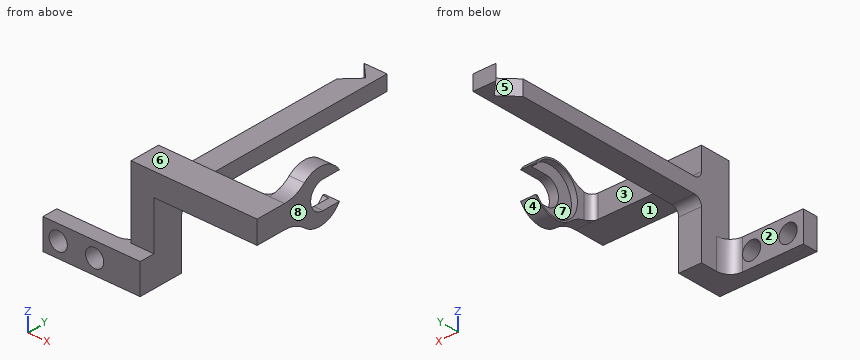
from build123d import *

# Parameters (mm, degrees)
SKETCH2_W                            = 22
SKETCH2_H                            = 10
SKETCH2_R                            = 3
BOSS_EXTRUDE1_DEPTH                  = 5
SKETCH3_W                            = 10
SKETCH3_H                            = 5
BOSS_EXTRUDE2_DEPTH                  = 10
BOSS_EXTRUDE3_DEPTH                  = 10
SKETCH5_W                            = 7.5
SKETCH5_H                            = 5
BOSS_EXTRUDE4_DEPTH                  = 75
CUT_EXTRUDE1_REACH                   = 98.857
BOSS_EXTRUDE5_DEPTH                  = 10
SKETCH13_W                           = 5
SKETCH13_H                           = 10
BOSS_EXTRUDE6_DEPTH                  = 7.5
BOSS_EXTRUDE7_DEPTH                  = 5
CUT_EXTRUDE5_REACH                   = 118.454
SKETCH16_R                           = 8
CUT_EXTRUDE6_DEPTH                   = 2
BOSS_EXTRUDE8_REACH                  = 104.314
BOSS_EXTRUDE8_END_RADIUS             = 11.091410312
BOSS_EXTRUDE8_DIRECTION_2_REACH      = 104.314
BOSS_EXTRUDE8_DIRECTION_2_END_RADIUS = 11.091410312
BOSS_EXTRUDE9_DEPTH                  = 7.5
BOSS_EXTRUDE10_START                 = -10
BOSS_EXTRUDE10_DEPTH                 = 10


with BuildPart() as part:
    # Sketch2 → Boss-Extrude1 (new body)
    with BuildSketch(Plane(origin=(0, 0, 0), x_dir=(1, 0, 0), z_dir=(0, 1, 0))):
        with Locations((6, 0)):
            Rectangle(SKETCH2_W, SKETCH2_H)
        with Locations(Location((0, 0, 0), (0, 0, 270))):
            Circle(SKETCH2_R, mode=Mode.SUBTRACT)
        with Locations(Location((12, 0, 0), (0, 0, 270))):
            Circle(SKETCH2_R, mode=Mode.SUBTRACT)
    extrude(amount=BOSS_EXTRUDE1_DEPTH)

    # Sketch3 → Boss-Extrude2 (add)
    with BuildSketch(Plane.XY.offset(5)):
        with Locations((22, 2.5)):
            Rectangle(SKETCH3_W, SKETCH3_H)
    extrude(amount=-BOSS_EXTRUDE2_DEPTH)

    # Sketch4 → Boss-Extrude3 (add)
    with BuildSketch(Plane(origin=(0, 5, 0), x_dir=(1, 0, 0), z_dir=(0, 1, 0))):
        Polygon((27, 5), (27, -5), (27, -7.5), (27, -18.5), (19.5, -18.5), (19.5, -7.5), (19.5, 5), align=None)
    extrude(amount=BOSS_EXTRUDE3_DEPTH)

    # Sketch5 → Boss-Extrude4 (add)
    with BuildSketch(Plane(origin=(0, 15, 0), x_dir=(1, 0, 0), z_dir=(0, 1, 0))):
        with Locations((23.25, -16)):
            Rectangle(SKETCH5_W, SKETCH5_H)
    extrude(amount=BOSS_EXTRUDE4_DEPTH)

    # Sketch6 → Cut-Extrude1 (cut, up to next)
    with BuildSketch(Plane.XY.offset(18.5), mode=Mode.PRIVATE) as cut_extrude1_sk1:
        Polygon((19.5, 90), (24.5, 85), (19.5, 80), align=None)
    cut_extrude1_tool1 = extrude(cut_extrude1_sk1.sketch, amount=-CUT_EXTRUDE1_REACH, mode=Mode.PRIVATE) & part.part
    add(cut_extrude1_tool1.solids().sort_by_distance((21.166667, 85, 18.5))[0], mode=Mode.SUBTRACT)

    # Sketch7 → Boss-Extrude5 (add)
    with BuildSketch(Plane(origin=(0, 15, 0), x_dir=(1, 0, 0), z_dir=(0, 1, 0))):
        Polygon((19.5, 5), (19.5, -28.5), (56, -28.5), (56, -21), (27, -21), (27, 5), align=None)
    extrude(amount=-BOSS_EXTRUDE5_DEPTH)

    # Sketch13 → Boss-Extrude6 (add)
    with BuildSketch(Plane(origin=(0, 0, 21), x_dir=(-1, 0, 0), z_dir=(0, 0, -1))):
        with Locations((-58.5, 10)):
            Rectangle(SKETCH13_W, SKETCH13_H)
    extrude(amount=-BOSS_EXTRUDE6_DEPTH)

    # Sketch14 → Boss-Extrude7 (add)
    with BuildSketch(Plane(origin=(61, 0, 0), x_dir=(0, 0, -1), z_dir=(1, 0, 0))):
        with BuildLine():
            Line((-29.25, 35), (-20.25, 35))
            ThreePointArc((-20.25, 35), (-16.346490099, 29.066011911), (-18.310852147, 22.240260236))
            ThreePointArc((-18.310852147, 22.240260236), (-20.306000981, 18.86176399), (-21, 15))
            Line((-21, 15), (-28.5, 15))
            ThreePointArc((-28.5, 15), (-29.193999019, 18.86176399), (-31.189147853, 22.240260236))
            ThreePointArc((-31.189147853, 22.240260236), (-33.153509901, 29.066011911), (-29.25, 35))
        make_face()
    extrude(amount=-BOSS_EXTRUDE7_DEPTH)

    # Sketch15 → Cut-Extrude5 (cut, up to next)
    with BuildSketch(Plane(origin=(61, 0, 0), x_dir=(0, 0, -1), z_dir=(1, 0, 0)), mode=Mode.PRIVATE) as cut_extrude5_sk1:
        with BuildLine():
            Line((-29.25, 35), (-29.25, 29))
            ThreePointArc((-29.25, 29), (-24.75, 24.5), (-20.25, 29))
            Line((-20.25, 29), (-20.25, 35))
            Line((-20.25, 35), (-29.25, 35))
        make_face()
    cut_extrude5_tool1 = extrude(cut_extrude5_sk1.sketch, amount=-CUT_EXTRUDE5_REACH, mode=Mode.PRIVATE) & part.part
    add(cut_extrude5_tool1.solids().sort_by_distance((61, 30.179951, 24.75))[0], mode=Mode.SUBTRACT)

    # Sketch16 → Cut-Extrude6 (cut)
    with BuildSketch(Plane(origin=(56, 0, 0), x_dir=(0, 0, -1), z_dir=(1, 0, 0))):
        with Locations((-24.75, 27.788897449)):
            Circle(SKETCH16_R)
    extrude(amount=CUT_EXTRUDE6_DEPTH, mode=Mode.SUBTRACT)

    # Boss-Extrude8: up to this cylinder (the profile starts outside it)
    boss_extrude8_end = Plane(origin=(55.44158, 15, 9.908589688), z_dir=(1, 0, 0)) * Cylinder(BOSS_EXTRUDE8_END_RADIUS, 231.810820624, mode=Mode.PRIVATE)
    # Sketch17 → Boss-Extrude8 (add, up to the surface)
    with BuildSketch(Plane(origin=(56, 15, 28.5), x_dir=(-1, 0, 0), z_dir=(0, 0, -1)), mode=Mode.PRIVATE) as boss_extrude8_sk1:
        with BuildLine():
            Line((0, 0), (0, 2.5))
            ThreePointArc((0, 2.5), (0.732233047, 0.732233047), (2.5, 0))
            Line((2.5, 0), (0, 0))
        make_face()
    boss_extrude8_tool1 = extrude(boss_extrude8_sk1.sketch, amount=BOSS_EXTRUDE8_REACH, mode=Mode.PRIVATE) - boss_extrude8_end
    add(boss_extrude8_tool1.solids().sort_by_distance((55.44158, 15.55842, 28.5))[0])

    # Boss-Extrude8 direction 2: up to this cylinder (the profile starts outside it)
    boss_extrude8_direction_2_end = Plane(origin=(55.44158, 15, 39.591410312), z_dir=(1, 0, 0)) * Cylinder(BOSS_EXTRUDE8_DIRECTION_2_END_RADIUS, 231.810820624, mode=Mode.PRIVATE)
    # Sketch17 → Boss-Extrude8 direction 2 (add, up to the surface)
    with BuildSketch(Plane(origin=(56, 15, 28.5), x_dir=(-1, 0, 0), z_dir=(0, 0, -1)), mode=Mode.PRIVATE) as boss_extrude8_direction_2_sk1:
        with BuildLine():
            Line((0, 0), (0, 2.5))
            ThreePointArc((0, 2.5), (0.732233047, 0.732233047), (2.5, 0))
            Line((2.5, 0), (0, 0))
        make_face()
    boss_extrude8_direction_2_tool1 = extrude(boss_extrude8_direction_2_sk1.sketch, amount=-BOSS_EXTRUDE8_DIRECTION_2_REACH, mode=Mode.PRIVATE) - boss_extrude8_direction_2_end
    add(boss_extrude8_direction_2_tool1.solids().sort_by_distance((55.44158, 15.55842, 28.5))[0])

    # Sketch18 → Boss-Extrude9 (add)
    with BuildSketch(Plane(origin=(27, 0, 0), x_dir=(0, 0, -1), z_dir=(1, 0, 0))):
        with BuildLine():
            Line((-13.5, 15), (-13.5, 17.5))
            ThreePointArc((-13.5, 17.5), (-12.767766953, 15.732233047), (-11, 15))
            Line((-11, 15), (-13.5, 15))
        make_face()
        with BuildLine():
            Line((-18.5, 15), (-18.5, 17.5))
            ThreePointArc((-18.5, 17.5), (-19.232233047, 15.732233047), (-21, 15))
            Line((-21, 15), (-18.5, 15))
        make_face()
    extrude(amount=-BOSS_EXTRUDE9_DEPTH)

    # Sketch19 → Boss-Extrude10 (add)
    with BuildSketch(Plane(origin=(0, 0, -5), x_dir=(-1, 0, 0), z_dir=(0, 0, -1)).offset(BOSS_EXTRUDE10_START)):
        with BuildLine():
            Line((-19.5, 5), (-19.5, 9.5))
            ThreePointArc((-19.5, 9.5), (-18.181980515, 6.318019485), (-15, 5))
            Line((-15, 5), (-19.5, 5))
        make_face()
    extrude(amount=BOSS_EXTRUDE10_DEPTH)


solid = part.part
Input: part model. Units: mm. Frame: model coordinates. Face numbers are marked on the shaded views. A direction names the side the tool comes from. Coordinates: 2 decimals unless noted, no trailing zeros. Loops run counter-clockwise (first coordinate to the right, second up) from the corner with the lowest first, then second, coordinate; pieces in that order, holes last.
(1) Section D-D on z = 24.75. Return the cut outline in (x, y), then the cut area to 3 significant figures.
(2) First-contact query: pin 1 Ø2.5 at (x, y) = (25, 52.5) entering from -Z; pin 2 Ø7.5 at (y, z) = (29.5, 28) entering from -X; pin 3 Ø6 at (x, z) = (24.5, 5) entering from +Y. Flat tips, straight axial feed; report the tip coordinate or a pass-through.
(3) Section C-C on x = 26. Return the cut outline in (y, z), then the cut area to 3 significant figures.
(4) Pull-direction query (X, two-part tool) for the marked faces 5, 6, 7 and 8; classes: released by +X, released by -X, zero draft, split by the parting line, or undercut.
(5) Set-up query: the marked faces 1, 2, 3 and 4. Return all of +Z, -Z, +X, -X, +Y, -Y with unobstructed straight access to the full face (end or side cutting, diameter ignored); none if empty.
(6) Section B-B on z = 1.5. Return the cut outline in (x, y), then the cut area to 3 significant figures.
(7) Section A-A on x = 12. Return the cut outline in (y, z), then the cut area to 3 significant figures.
(8) Material intervals for probe 1 along X at (y, z) = (2.45, 0); probe 2 along Z at (x, y) = (12, 2.1); probe 3 along Z at (x, y) = (40, 5.5), sorted ascending.
Data:
1. outline: (19.5, 5) - (61, 5) - (61, 24.5) - (58, 24.5) - (58, 19.79) - (56, 19.79) - (56, 17.5) arc R2.5 cw to (53.5, 15) - (19.5, 15) - close
1. area: 454 mm2
2. pin 1: stops at z = 13.5
2. pin 2: stops at x = 58
2. pin 3: stops at y = 15
3. outline: (0, -5) - (15, -5) - (15, 11) arc R2.5 cw to (17.5, 13.5) - (90, 13.5) - (90, 18.5) - (17.5, 18.5) arc R2.5 cw to (15, 21) - (15, 28.5) - (5, 28.5) - (5, 5) - (0, 5) - close
3. area: 763 mm2
4. face 5: released by -X
4. face 6: zero draft
4. face 7: undercut
4. face 8: released by +X
5. face 1: -Z, +X, -Y
5. face 2: +Z, -Z, -X, +Y
5. face 3: +Z, -X, +Y
5. face 4: -Z, +X
6. outline: (-5, 0) - (-2.6, 0) - (-2.6, 5) - (-5, 5) - close; (2.6, 0) - (9.4, 0) - (9.4, 5) - (2.6, 5) - close; (14.6, 0) - (27, 0) - (27, 15) - (19.5, 15) - (19.5, 9.5) arc R4.5 cw to (15, 5) - (14.6, 5) - close
6. area: 187 mm2
7. outline: (0, -5) - (5, -5) - (5, -3) - (0, -3) - close; (0, 3) - (5, 3) - (5, 5) - (0, 5) - close
7. area: 20.0 mm2
8. probe 1: x = -5 to -3, 3 to 9, 15 to 27
8. probe 2: z = -5 to -3, 3 to 5
8. probe 3: z = 21 to 28.5
